The model under review builds one solid part; all positions refer to its coordinate system, in mm. A direction names the side the tool comes from. Round coordinates to 2 decimals unless told otherwise and drop trailing zeros. Write each loop counter-clockwise with the first axis right and the second up, starting at its lowest first coordinate (ties: lowest second). Pieces come first, ordered by that corner, then holes. Notation, with made-up numbers: M -34.5,-34.5 L -14.5,-34.5 A24 cw -14.5,-10.5 Z; hole C 33.25,-33 d8. An arc over 180 degrees is marked long. Write item = value, one per line. Start each with the question number.
Item 1: To check wall thickness, follow line 1 along Z through (x, y) = (14.75, -116) (3 decimals); line 2 along X through (y, z) = (128, 2.75). State the ranges of each line that lie inside material, in increasing order.
Item 2: Take a section at C-C, the plane z = 10.25. Give the boundary of the cut face in (x, y) (3 decimals), plus the area to 3 significant figures.
Item 3: Tool access review of faces 1 (the flat face through (10, -3, 3.175)), 2 (the flat face through (3, -228.6, 7)): name each direction out of +Z, -Z, +X, -X, +Y, -Y from which nothing blocks a thin tool from reaching the whole face with its end or side.
Item 4: Take a section at A-A, the plane y = 193.5. Give the boundary of the cut face in (x, z) (3 decimals).
Item 5: For pin 1 Ø4 at (x, z) = (6.5, 12.5) entering from +Y; pin 2 Ø5 at (x, y) = (12.5, -30) entering from +Z (3 decimals); pin 3 Ø10 at (y, z) = (21, 11) entering from +X (3 decimals); pin 4 Ø8 at (x, y) = (6.5, -64) entering from +Z, all flat-tipped, find the tip position at first contact; note any pin that passes through.
Item 6: Take a section at B-B, the plane x = 12.25. Give the boundary of the cut face in (y, z) (3 decimals).
from build123d import *

# Parameters (mm, degrees)
F1_DEPTH = 228.6


with BuildPart() as f1:
    # F0 (on Front) → F1 (new body, symmetric)
    with BuildSketch(Plane.XZ):
        with BuildLine():
            ThreePointArc((3.175, 15.875), (2.245064, 18.120064), (0, 19.05))
            Line((0, 19.05), (0, 0))
            Line((0, 0), (19.05, 0))
            ThreePointArc((19.05, 0), (18.120064, 2.245064), (15.875, 3.175))
            Line((15.875, 3.175), (3.175, 3.175))
            Line((3.175, 3.175), (3.175, 15.875))
        make_face()
    extrude(amount=F1_DEPTH, both=True)


solid = f1.part
Response values:
q1.line_1 = 0 to 3.175
q1.line_2 = 0 to 17.46
q2.outline = M 0,-228.6 L 3.175,-228.6 L 3.175,228.6 L 0,228.6 Z
q2.area = 1,450 mm2
q3.face_1 = +Z, +X, +Y, -Y
q3.face_2 = +Z, -Z, +X, -X, -Y
q4.outline = M 0,0 L 19.05,0 A3.175 ccw 15.875,3.175 L 3.175,3.175 L 3.175,15.875 A3.175 ccw 0,19.05 Z
q5.pin_1 = through
q5.pin_2 = 3.175
q5.pin_3 = 3.175
q5.pin_4 = 17.83
q6.outline = M -228.6,0 L 228.6,0 L 228.6,3.175 L -228.6,3.175 Z
